Check sheet for the modelled part. Datum: model origin and axes. Units: mm. A direction names the side the tool comes from. Give positions to 0.01 mm unless a question says otherwise; leave off trailing zeros. Order: outer loops, then holes, each group sorted by start corner. A loop starts at its lowest first (then second) coordinate and runs counter-clockwise, first axis right, second up. Notation, with made-up numbers: M 53,58.25 L 79,58.25 A26 ccw 79,75.25 Z; hole C 85.5,-32.5 d9. An arc over 180 degrees is marked long. One line per question, with ' | ' between items. Start each with the question number.
```python
from build123d import *

# Parameters (mm, degrees)
F0_W     = 19.05
F0_H     = 609.6
F1_DEPTH = 533.4
F2_W     = 19.05
F2_H     = 50.8
F3_DEPTH = 19.05
F4_W     = 19.05
F4_H     = 50.8
F5_DEPTH = 19.05
F6_R     = 25.4
F7_DEPTH = 19.05


with BuildPart() as f1:
    # F0 (on Top) → F1 (new body)
    with BuildSketch(Plane.XY):
        with Locations((9.525, 304.8)):
            Rectangle(F0_W, F0_H)
    extrude(amount=F1_DEPTH)

    # F2 (on face) → F3 (join)
    with BuildSketch(Plane(origin=(0, 0, 0), x_dir=(1, 0, 0), z_dir=(0, 0, -1))):
        with Locations((9.525, -152.4)):
            Rectangle(F2_W, F2_H)
        with Locations((9.525, -273.05)):
            Rectangle(F2_W, F2_H)
        with Locations((9.525, -393.7)):
            Rectangle(F2_W, F2_H)
        with Locations((9.525, -514.35)):
            Rectangle(F2_W, F2_H)
    extrude(amount=F3_DEPTH)

    # F4 (on face) → F5 (join)
    with BuildSketch(Plane.XY.offset(533.4)):
        with Locations((9.525, 514.35)):
            Rectangle(F4_W, F4_H)
        with Locations((9.525, 393.7)):
            Rectangle(F4_W, F4_H)
        with Locations((9.525, 273.05)):
            Rectangle(F4_W, F4_H)
        with Locations((9.525, 152.4)):
            Rectangle(F4_W, F4_H)
    extrude(amount=F5_DEPTH)

    # F6 (on face) → F7 (cut)
    with BuildSketch(Plane(origin=(0, 0, 0), x_dir=(0, -1, 0), z_dir=(-1, 0, 0))):
        with Locations((-488.95, 101.6)):
            Circle(F6_R)
        with Locations((-368.3, 101.6)):
            Circle(F6_R)
        with Locations((-247.65, 101.6)):
            Circle(F6_R)
        with Locations((-127, 101.6)):
            Circle(F6_R)
        with Locations((-488.95, 431.8)):
            Circle(F6_R)
        with Locations((-368.3, 431.8)):
            Circle(F6_R)
        with Locations((-247.65, 431.8)):
            Circle(F6_R)
        with Locations((-127, 431.8)):
            Circle(F6_R)
        with Locations((-127, 266.7)):
            Circle(F6_R)
        with Locations((-488.95, 266.7)):
            Circle(F6_R)
    extrude(amount=-F7_DEPTH, mode=Mode.SUBTRACT)


solid = f1.part
```
Item 1: Section check A-A, the plane z = 431.8. Record the cut outline in (x, y).
Item 2: Scan lines: probe 1 along Z at (x, y) = (4, 267); probe 2 along Y at (x, z) = (2.5, 246); probe 3 along Z at (x, y) = (14.5, 387). Record each from-to range of solid material in increasing order. Write a range as [from, to].
Item 3: Section check B-B, the plane z = 266.7. Record the cut outline in (x, y), then the cut area to 3 significant figures.
Item 4: Set-up check for faces 1 (the face through (9, 455, 0)), 2 (the face through (9, 488.95, 543)), 3 (the face through (9, 127, -9)), 4 (the face through (9, 127, 543)): record each of +Z, -Z, +X, -X, +Y, -Y from which the full face is reachable in a straight line by a thin tool's end or side.
Item 5: Section check C-C, the plane y = 321. Record the cut outline in (x, z).
Item 6: Section check D-D, the plane x = 8.75. State how many separate pieces and enclosed holes the cut face has, then the cut area to 3 significant figures.
Item 7: Go/stop test with flat-tipped pins: P1, Ø5.5, axis at x = 13, z = -12, coming from the +Y side; P2, Ø9.5, axis at x = 7, z = -12, coming from the -Y side; P3, Ø10, axis at x = 17, y = 450.5, coming from the -Z side. Record where each tip stops, or that it passes through.
Reported:
1) outline: M 0,0 L 19.05,0 L 19.05,101.6 L 0,101.6 Z; M 0,152.4 L 19.05,152.4 L 19.05,222.25 L 0,222.25 Z; M 0,273.05 L 19.05,273.05 L 19.05,342.9 L 0,342.9 Z; M 0,393.7 L 19.05,393.7 L 19.05,463.55 L 0,463.55 Z; M 0,514.35 L 19.05,514.35 L 19.05,609.6 L 0,609.6 Z
2) probe 1: z = [-19.05, 85.15], [118.05, 415.35], [448.25, 552.45] | probe 2: y = [0, 112.28], [141.72, 474.23], [503.67, 609.6] | probe 3: z = [-19.05, 84.41], [118.79, 414.61], [448.99, 552.45]
3) outline: M 0,0 L 19.05,0 L 19.05,101.6 L 0,101.6 Z; M 0,152.4 L 19.05,152.4 L 19.05,463.55 L 0,463.55 Z; M 0,514.35 L 19.05,514.35 L 19.05,609.6 L 0,609.6 Z | area: 9,680 mm^2
4) face 1: -Z, +X, -X | face 2: +Z, +X, -X | face 3: -Z, +X, -X, -Y | face 4: +Z, +X, -X, -Y
5) outline: M 0,0 L 19.05,0 L 19.05,533.4 L 0,533.4 Z
6) separate pieces: 1 | enclosed holes: 10 | area: 313,000 mm^2
7) P1: stops at y = 539.75 | P2: stops at y = 127 | P3: stops at z = 0
